Input: part model. Units: mm. Frame: model coordinates. A direction names the side the tool comes from. Coordinates: 2 decimals unless noted, no trailing zeros. Write each loop counter-clockwise with the first axis right and the second up, starting at its lowest first coordinate (ties: lowest second). Pieces come first, ordered by that corner, then holes. Notation, with made-up numbers: (-6.5, 43.5) - (50.5, 43.5) arc R21 ccw to (50.5, 68.5) - close; hole circle Ø3 at (84.25, 5.25). An arc over 180 degrees is marked (long way). Use CSV: the item, a comma, the result in double quotes.
```python
from build123d import *

# Parameters (mm, degrees)
RESSALTO_EXTRUS_O1_DEPTH = 5
ESBO_O2_W                = 7
ESBO_O2_H                = 10
RESSALTO_EXTRUS_O2_DEPTH = 20
ESBO_O4_R                = 1.5
CORTE_EXTRUS_O1_DEPTH    = 98.269963506
ESBO_O5_W                = 5
ESBO_O5_H                = 40
RESSALTO_EXTRUS_O3_DEPTH = 7


with BuildPart() as part:
    # Esboço1 → Ressalto-extrusão1 (new body)
    with BuildSketch(Plane(origin=(0, 0, 0), x_dir=(1, 0, 0), z_dir=(0, 1, 0))):
        with BuildLine():
            Line((-13.214501511, 15.533232628), (79.785498489, 15.533232628))
            ThreePointArc((79.785498489, 15.533232628), (86.856566301, 12.60430044), (89.785498489, 5.533232628))
            Line((89.785498489, 5.533232628), (89.785498489, -34.466767372))
            ThreePointArc((89.785498489, -34.466767372), (86.856566301, -41.537835183), (79.785498489, -44.466767372))
            Line((79.785498489, -44.466767372), (-13.214501511, -44.466767372))
            ThreePointArc((-13.214501511, -44.466767372), (-20.285569322, -41.537835183), (-23.214501511, -34.466767372))
            Line((-23.214501511, -34.466767372), (-23.214501511, 5.533232628))
            ThreePointArc((-23.214501511, 5.533232628), (-20.285569322, 12.60430044), (-13.214501511, 15.533232628))
        make_face()
    extrude(amount=RESSALTO_EXTRUS_O1_DEPTH)

    # Esboço2 → Ressalto-extrusão2 (add)
    with BuildSketch(Plane(origin=(0, 5, 0), x_dir=(1, 0, 0), z_dir=(0, 1, 0))):
        with Locations((56.105498489, -4.747557162)):
            Rectangle(ESBO_O2_W, ESBO_O2_H)
        with Locations((10.465498489, -4.747557162)):
            Rectangle(ESBO_O2_W, ESBO_O2_H)
    extrude(amount=RESSALTO_EXTRUS_O2_DEPTH)

    # Esboço4 → Corte-extrusão1 (cut, through all)
    with BuildSketch(Plane.ZY.offset(-6.965498489)):
        with Locations((4.747557162, 15)):
            Circle(ESBO_O4_R)
    extrude(amount=-CORTE_EXTRUS_O1_DEPTH, mode=Mode.SUBTRACT)

    # Esboço5 → Ressalto-extrusão3 (add)
    with BuildSketch(Plane(origin=(0, 5, 0), x_dir=(1, 0, 0), z_dir=(0, 1, 0))):
        with Locations((-12.714501511, -14.466767372)):
            Rectangle(ESBO_O5_W, ESBO_O5_H)
        with Locations((79.285498489, -14.466767372)):
            Rectangle(ESBO_O5_W, ESBO_O5_H)
    extrude(amount=RESSALTO_EXTRUS_O3_DEPTH)


solid = part.part
```
(1) Cut plane A-A on y = 15. Return loops of the section in (x, z).
Check values:
outline,"(6.97, -0.25) - (13.97, -0.25) - (13.97, 3.25) - (6.97, 3.25) - close; (6.97, 6.25) - (13.97, 6.25) - (13.97, 9.75) - (6.97, 9.75) - close; (52.61, -0.25) - (59.61, -0.25) - (59.61, 3.25) - (52.61, 3.25) - close; (52.61, 6.25) - (59.61, 6.25) - (59.61, 9.75) - (52.61, 9.75) - close"
(2) Cut plane C-C on z = -9.5. Return loops of the section in (x, y), and give its area (3 significant figures).
Check values:
outline,"(-22.39, 0) - (88.97, 0) - (88.97, 5) - (-22.39, 5) - close"
area,"557 mm^2"
(3) Cut plane B-B on x = 31.5. Return loops of the section in (y, z).
Check values:
outline,"(0, -15.53) - (5, -15.53) - (5, 44.47) - (0, 44.47) - close"
(4) Pin query (flat end, axial travel): pin 1 Ø12 at (x, z) = (-4.5, 35) entering from +Y; pin 2 Ø4 at (x, y) = (78, 8.5) entering from +Z; pin 3 Ø11 at (y, z) = (14.5, 3) entering from +X. Return the tip coordinate at first contact, or that it passes through.
Check values:
pin 1,"y = 12"
pin 2,"z = 34.47"
pin 3,"x = 81.79"
(5) Ray query, probe 1 along X at (y, z) = (8.5, 14); probe 2 along Y at (x, z) = (-16, 15.5); probe 3 along Y at (x, z) = (79, 25). Return the intervals inside material, ascending. Write a range as from..to.
Check values:
probe 1,"-15.21..-10.21, 76.79..81.79"
probe 2,"0..5"
probe 3,"0..12"
(6) Reachability of faces 4 (the flat face through (79, 8, -5.533)), 5 (the flat face through (56, 15, 9.748)), 6 (the flat face through (-15.215, 8, 15)), 7 (the flat face through (-13, 8, 34.467)) from +Z, -Z, +X, -X, +Y, -Y: full face, straight path, thin tool, end or side. Return the list, or none.
Check values:
face 4,"-Z, +X, -X, +Y"
face 5,"+Z, +Y"
face 6,"+Z, -Z, -X, +Y"
face 7,"+Z, +X, -X, +Y"
(7) Draft query along X for faces 1 (the cylindrical face through (86.934, 2.465, 41.46)), 2 (the flat face through (6.965, 15, 3)), 3 (the flat face through (-13, 8, -5.533)). Return one class per face: pulls with the +X half, pulls with the -X half, needs draft (parallel to the pull), parting line crosses it, or undercut.
Check values:
face 1,"pulls with the +X half"
face 2,"undercut"
face 3,"needs draft"
